from build123d import *

# Parameters (mm, degrees)
F1_DEPTH = 19.05
F2_DEPTH = 152.4
F3_DEPTH = 152.4
F4_DEPTH = 146.05


with BuildPart() as f1:
    # F0 (on Top) → F1 (new body)
    with BuildSketch(Plane.XY):
        with BuildLine():
            Line((-596.9, 871.074308), (-596.9, -906.925692))
            Line((-596.9, -906.925692), (0, -906.925692))
            Line((0, -906.925692), (0, -30.625692))
            ThreePointArc((0, -30.625692), (89.273853, 184.900455), (304.8, 274.174308))
            Line((304.8, 274.174308), (1181.1, 274.174308))
            Line((1181.1, 274.174308), (1181.1, 871.074308))
            Line((1181.1, 871.074308), (-596.9, 871.074308))
        make_face()
        Polygon((-539.75, 190.08354), (-539.75, 813.924308), (84.090768, 813.924308), align=None, mode=Mode.SUBTRACT)
        Polygon((-520.7, 794.874308), (-520.7, 236.074308), (38.1, 794.874308), align=None)
        Polygon((84.090768, 813.924308), (-539.75, 813.924308), (-539.75, 190.08354), align=None)
        Polygon((38.1, 794.874308), (-520.7, 236.074308), (-520.7, 794.874308), align=None, mode=Mode.SUBTRACT)
    extrude(amount=-F1_DEPTH)

    # F0 (on Top) → F2 (join)
    with BuildSketch(Plane.XY):
        Polygon((84.090768, 813.924308), (-539.75, 813.924308), (-539.75, 190.08354), align=None)
        Polygon((38.1, 794.874308), (-520.7, 236.074308), (-520.7, 794.874308), align=None, mode=Mode.SUBTRACT)
    extrude(amount=-F2_DEPTH)

    # F0 (on Top) → F3 (join)
    with BuildSketch(Plane.XY):
        Polygon((-520.7, 794.874308), (-520.7, 236.074308), (38.1, 794.874308), align=None)
    extrude(amount=-F3_DEPTH)

    # F0 (on Top) → F4 (cut)
    with BuildSketch(Plane.XY):
        Polygon((-520.7, 794.874308), (-520.7, 236.074308), (38.1, 794.874308), align=None)
    extrude(amount=-F4_DEPTH, mode=Mode.SUBTRACT)


solid = f1.part
Check sheet for the modelled part. Datum: model origin and axes. Units: mm. A direction names the side the tool comes from. Round coordinates to 2 decimals unless told otherwise and drop trailing zeros. Loops run counter-clockwise (first coordinate to the right, second up) from the corner with the lowest first, then second, coordinate; pieces in that order, holes last.
1. Sectioned sample at B-B on x = -121.5. Record the boundary of the cut face in (y, z).
2. Sectioned sample at A-A on z = -87. Record the boundary of the cut face in (x, y).
3. Mould release check, pull along Y, two halves, no side actions. Record for faces 1 (the flat face through (-307, 581, -146.05)), 2 (the cylindrical face through (86.9, 182.5, -9.4)), 3 (the flat face through (-223, 813.924, -85)), 4 (the flat face through (82, 192, -19.05)): released by +Y, released by -Y, zero draft, split by the parting line, or undercut.
4. Sectioned sample at C-C on y = 423.5. Record the boundary of the cut face in (x, z), and give its area (3 significant figures).
5. Sectioned sample at D-D on x = 952.5. Record the boundary of the cut face in (y, z), and give its area (3 significant figures).
6. Set-up check for faces 5 (the flat face through (-232.197, 497.637, -84.792)), 6 (the flat face through (-539.75, 506, -85)), 7 (the flat face through (-302, 576, -152.4)), 8 (the flat face through (-520.7, 519, -72)): record each of +Z, -Z, +X, -X, +Y, -Y from which the full face is reachable in a straight line by a thin tool's end or side.
7. Gauge pin test, flat ends, axial feed: pin 1 Ø15 at (x, z) = (856.5, -5.5) entering from -Y; pin 2 Ø5.5 at (y, z) = (-512.5, -7) entering from +X; pin 3 Ø12 at (y, z) = (588, -112.5) entering from +X; pin 4 Ø10 at (y, z) = (418, -23) entering from -X. Record the tip position at first contact, or that the pin passes through.
8. Scan lines: probe 1 along Z at (x, y) = (-468.5, -129); probe 2 along Y at (x, z) = (-421, -44.5); probe 3 along Y at (x, z) = (-427, -97). Record each from-to range of solid material in increasing order.
Recorded:
1. outline: (-906.93, -19.05) - (608.33, -19.05) - (608.33, -152.4) - (813.92, -152.4) - (813.92, -19.05) - (871.07, -19.05) - (871.07, 0) - (794.87, 0) - (794.87, -146.05) - (635.27, -146.05) - (635.27, 0) - (-906.93, 0) - close
2. outline: (-539.75, 190.08) - (84.09, 813.92) - (-539.75, 813.92) - close; hole (-520.7, 236.07) - (38.1, 794.87) - (-520.7, 794.87) - close
3. face 1: undercut
3. face 2: released by -Y
3. face 3: released by +Y
3. face 4: zero draft
4. outline: (-596.9, -19.05) - (-539.75, -19.05) - (-539.75, -152.4) - (-306.33, -152.4) - (-306.33, -19.05) - (1181.1, -19.05) - (1181.1, 0) - (-333.27, 0) - (-333.27, -146.05) - (-520.7, -146.05) - (-520.7, 0) - (-596.9, 0) - close
4. area: 37,600 mm2
5. outline: (274.17, -19.05) - (871.07, -19.05) - (871.07, 0) - (274.17, 0) - close
5. area: 11,400 mm2
6. face 5: -Z, +X, -Y
6. face 6: -Z, -X, +Y, -Y
6. face 7: -Z, +X, -X, +Y, -Y
6. face 8: +Z
7. pin 1: stops at y = 274.17
7. pin 2: stops at x = 0
7. pin 3: stops at x = -135.83
7. pin 4: stops at x = -596.9
8. probe 1: z = -19.05 to 0
8. probe 2: y = 308.83 to 335.77, 794.87 to 813.92
8. probe 3: y = 302.83 to 329.77, 794.87 to 813.92
